Part model, mm, in its own coordinate system. Face numbers are marked on the shaded views. A direction names the side the tool comes from. Coordinates: 2 decimals unless noted, no trailing zeros. Order: outer loops, then holes, each group sorted by start corner. A loop starts at its lowest first (then second) coordinate and runs counter-clockwise, first axis right, second up.
1) Cut at C-C (z = -1.5). Give the number of separate pieces and of enclosed holes in the cut face, and give its area (3 significant figures).
2) Wall check: L1, parallel to X at y = 17.5, z = 7; L2, parallel to X at y = 3.7, z = 15.5; L3, parallel to Y at x = 15.8, z = 0. Give the ranges that are in metal, low to high.
3) Cut at A-A (y = 11.75). List the corners of the cut face in (x, z).
4) Cut at D-D (y = 18.75). List the corners of the cut face in (x, z).
5) Cut at B-B (x = -1). List the corners of the cut face in (y, z).
6) Tool access for the marked faces 1, 2, 3 and 4: list every direction of +Z, -Z, +X, -X, +Y, -Y with a clear straight run to the whole face (end or side of a thin tool).
7) Pin check, flat tips, straight feed: pin 1 Ø2 at (y, z) = (10.5, -8.5) entering from +X; pin 2 Ø4 at (x, y) = (18, 12.5) entering from -Z; pin 3 Ø1.6 at (x, z) = (20.5, 2) entering from +Y; pin 4 Ø10 at (x, y) = (-5.5, 15.5) entering from +Z. Stop position of each tip, or through.
8) Mould opens along X. For the marked faces 5, 6 and 7 say: +X half, -X half, draft (parallel to the pull), parting line (faces both ways), or undercut.
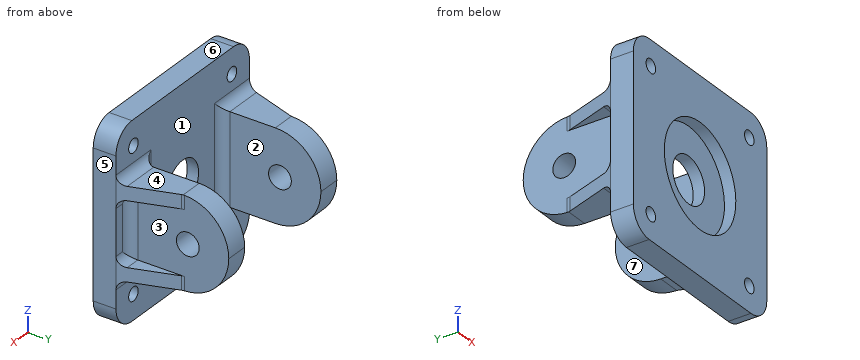
```python
from build123d import *

# Parameters (mm, degrees)
SKETCH1_W               = 42
SKETCH1_H               = 42
SKETCH1_R               = 1.5
BOSS_EXTRUDE1_DEPTH     = 5
SKETCH2_W               = 5
SKETCH2_H               = 20
BOSS_EXTRUDE2_DEPTH     = 27
CUT_EXTRUDE1_DEPTH      = 41.137264481
CUT_EXTRUDE1_DEPTH_BACK = 41.137264481
SKETCH3_R               = 2.5
FILLET1_R               = 10
FILLET2_R               = 5
SKETCH4_R               = 11.25
CUT_EXTRUDE2_DEPTH      = 2.5
SKETCH5_R               = 5
CUT_EXTRUDE3_DEPTH      = 10
SKETCH6_W               = 4
SKETCH6_H               = 3
BOSS_EXTRUDE3_DEPTH     = 17
CUT_EXTRUDE4_DEPTH      = 41.137264481
CUT_EXTRUDE4_DEPTH_BACK = 41.137264481
FILLET3_R               = 2


with BuildPart() as part:
    # Sketch1 → Boss-Extrude1 (new body)
    with BuildSketch(Plane(origin=(0, 0, 0), x_dir=(1, 0, 0), z_dir=(0, 1, 0))):
        Rectangle(SKETCH1_W, SKETCH1_H)
        with Locations(Location((-15.5, 15.5, 0), (0, 0, 270))):
            Circle(SKETCH1_R, mode=Mode.SUBTRACT)
        with Locations(Location((15.5, 15.5, 0), (0, 0, 270))):
            Circle(SKETCH1_R, mode=Mode.SUBTRACT)
        with Locations(Location((15.5, -15.5, 0), (0, 0, 270))):
            Circle(SKETCH1_R, mode=Mode.SUBTRACT)
        with Locations(Location((-15.5, -15.5, 0), (0, 0, 270))):
            Circle(SKETCH1_R, mode=Mode.SUBTRACT)
    extrude(amount=BOSS_EXTRUDE1_DEPTH)

    # Sketch2 → Boss-Extrude2 (add)
    with BuildSketch(Plane(origin=(0, 0, 0), x_dir=(1, 0, 0), z_dir=(0, 1, 0))):
        with Locations((-14.5, 0)):
            Rectangle(SKETCH2_W, SKETCH2_H)
        with Locations((14.5, 0)):
            Rectangle(SKETCH2_W, SKETCH2_H)
    extrude(amount=BOSS_EXTRUDE2_DEPTH)

    # Sketch3 → Cut-Extrude1 (cut, two sides: drawn at the far end of the back side and taken through both)
    with BuildSketch(Plane(origin=(0, 0, 0), x_dir=(0, 0, -1), z_dir=(1, 0, 0)).offset(-CUT_EXTRUDE1_DEPTH_BACK)):
        with Locations((0, 18)):
            Circle(SKETCH3_R)
    extrude(amount=CUT_EXTRUDE1_DEPTH + CUT_EXTRUDE1_DEPTH_BACK, mode=Mode.SUBTRACT)

    # Fillet1
    fillet1_edges = [part.edges().sort_by_distance(p)[0] for p in [
        (-14.5, 27, 10),
        (-14.5, 27, -10),
        (14.5, 27, -10),
        (14.5, 27, 10),
    ]]
    fillet(fillet1_edges, radius=FILLET1_R - 0.0001)  # a hair under: the kernel refuses the full size

    # Fillet2
    fillet2_edges = [part.edges().sort_by_distance(p)[0] for p in [
        (21, 2.5, 21),
        (-21, 2.5, 21),
        (-21, 2.5, -21),
        (21, 2.5, -21),
    ]]
    fillet(fillet2_edges, radius=FILLET2_R)

    # Sketch4 → Cut-Extrude2 (cut)
    with BuildSketch(Plane(origin=(0, 0, 0), x_dir=(1, 0, 0), z_dir=(0, 1, 0))):
        with Locations(Location((0, 0, 0), (0, 0, 270))):
            Circle(SKETCH4_R)
    extrude(amount=CUT_EXTRUDE2_DEPTH, mode=Mode.SUBTRACT)

    # Sketch5 → Cut-Extrude3 (cut)
    with BuildSketch(Plane(origin=(0, 0, 0), x_dir=(1, 0, 0), z_dir=(0, 1, 0))):
        with Locations(Location((0, 0, 0), (0, 0, 270))):
            Circle(SKETCH5_R)
    extrude(amount=CUT_EXTRUDE3_DEPTH, mode=Mode.SUBTRACT)

    # Sketch6 → Boss-Extrude3 (add)
    with BuildSketch(Plane(origin=(0, 0, 0), x_dir=(1, 0, 0), z_dir=(0, 1, 0))):
        with Locations((-19, 8.5)):
            Rectangle(SKETCH6_W, SKETCH6_H)
        with Locations((-19, -8.5)):
            Rectangle(SKETCH6_W, SKETCH6_H)
        with Locations((19, -8.5)):
            Rectangle(SKETCH6_W, SKETCH6_H)
        with Locations((19, 8.5)):
            Rectangle(SKETCH6_W, SKETCH6_H)
    extrude(amount=BOSS_EXTRUDE3_DEPTH)

    # Sketch7 → Cut-Extrude4 (cut, two sides: drawn at the far end of the back side and taken through both)
    with BuildSketch(Plane.XY.offset(-CUT_EXTRUDE4_DEPTH_BACK)):
        Polygon((-17, 17), (-21, 5), (-21, 17), align=None)
        Polygon((17, 17), (21, 17), (21, 5), align=None)
    extrude(amount=CUT_EXTRUDE4_DEPTH + CUT_EXTRUDE4_DEPTH_BACK, mode=Mode.SUBTRACT)

    # Fillet3
    fillet3_edges = [part.edges().sort_by_distance(p)[0] for p in [
        (-19, 5, -7),
        (-17, 17, -8.5),
        (-17, 5, 0),
        (-19, 5, 7),
        (-17, 17, 8.5),
        (19, 5, 7),
        (17, 17, 8.5),
        (17, 5, 0),
        (19, 5, -7),
        (17, 17, -8.5),
        (-16.5, 5, 10),
        (-12, 5, 0),
        (-16.5, 5, -10),
        (16.5, 5, -10),
        (12, 5, 0),
        (16.5, 5, 10),
    ]]
    fillet(fillet3_edges, radius=FILLET3_R)


solid = part.part
```
Geometry check:
1. separate pieces: 4
1. enclosed holes: 0
1. area: 313 mm2
2. L1: x = -17 to -12, 12 to 17
2. L2: x = -21 to -17, -14 to 14, 17 to 21
2. L3: y = 0 to 15.5, 20.5 to 27
3. outline: (-18.75, -10) - (-12, -10) - (-12, 10) - (-18.75, 10) - (-18.75, 7) - (-17, 7) - (-17, -7) - (-18.75, -7) - close; (12, -10) - (18.75, -10) - (18.75, -7) - (17, -7) - (17, 7) - (18.75, 7) - (18.75, 10) - (12, 10) - close
4. outline: (-17, -9.85) - (-12, -9.85) - (-12, -2.38) - (-17, -2.38) - close; (-17, 2.38) - (-12, 2.38) - (-12, 9.85) - (-17, 9.85) - close; (12, -9.85) - (17, -9.85) - (17, -2.38) - (12, -2.38) - close; (12, 2.38) - (17, 2.38) - (17, 9.85) - (12, 9.85) - close
5. outline: (0, -21) - (5, -21) - (5, -4.9) - (2.5, -4.9) - (2.5, -11.21) - (0, -11.21) - close; (0, 11.21) - (2.5, 11.21) - (2.5, 4.9) - (5, 4.9) - (5, 21) - (0, 21) - close
6. face 1: +Y
6. face 2: +Z, -Z, +Y
6. face 3: +X, +Y
6. face 4: +Z, +X, -X, +Y
7. pin 1: stops at x = 19.5
7. pin 2: stops at z = -10
7. pin 3: stops at y = 5
7. pin 4: passes through
8. face 5: +X half
8. face 6: draft
8. face 7: undercut
